from build123d import *

# Parameters (mm, degrees)
F0_W     = 10
F0_H     = 8
F1_DEPTH = 10
F2_T     = 1
F3_W     = 8
F3_H     = 2.908741124
F4_DEPTH = 0.1


with BuildPart() as f1:
    # F0 (on Top) → F1 (new body)
    with BuildSketch(Plane.XY):
        with Locations((-44.9863001704, 1.6067679121)):
            Rectangle(F0_W, F0_H)
    extrude(amount=F1_DEPTH)

    # F2
    f2_openings = [f1.faces().sort_by_distance(p)[0] for p in [
        (-44.9863, 1.606768, 10),
    ]]
    offset(amount=F2_T, openings=f2_openings, kind=Kind.INTERSECTION)

    # F3 (on face) → F4 (join)
    with BuildSketch(Plane.YZ.offset(-38.9863001704)):
        with Locations((1.6067679121, 6.545629438)):
            Rectangle(F3_W, F3_H)
    extrude(amount=F4_DEPTH)


solid = f1.part
For this review, take the finished solid that the model builds, in its own axes (mm). A direction names the side the tool comes from. Round coordinates to 2 decimals unless told otherwise and drop trailing zeros. Loops run counter-clockwise (first coordinate to the right, second up) from the corner with the lowest first, then second, coordinate; pieces in that order, holes last. Notation, with made-up numbers: (18, -24) - (25, -24) arc R20 cw to (25, 8) - close; hole circle Ø8 at (52, 35.5). An arc over 180 degrees is marked (long way). Use one line per item in the form item = value.
1) Mouldability with a two-part tool opening along Y and no side actions: class faces 3 (the face through (-39.986, 2, 5)), 4 (the face through (-50.986, 2, 4)), 5 (the face through (-45, 6.607, 4)) as pulls with the +Y half, pulls with the -Y half, needs draft (parallel to the pull), parting line crosses it, or undercut.
Solutions:
face_3 = undercut
face_4 = needs draft
face_5 = pulls with the +Y half
2) Clearance check with flat-ended pins moving along their axes: P1, Ø2, axis at x = -46, y = 2.5, coming from the +Z side; P2, Ø5, axis at y = 4, z = 2, coming from the +X side. State where each tip first meets the part, or that it passes through.
Solutions:
P1 = 0
P2 = -38.99
3) Wall thickness on probe 1 along Y at (x, z) = (-49, 5.25); probe 2 along X at (y, z) = (1.5, 2); probe 3 along X at (y, z) = (4, 6.25): over which ranges is each line inside the solid? List them lowest first.
Solutions:
probe_1 = -3.39 to -2.39, 5.61 to 6.61
probe_2 = -50.99 to -49.99, -39.99 to -38.99
probe_3 = -50.99 to -49.99, -39.99 to -38.89
4) We need section C-C on x = -43.5. Write out the cut boundary in (y, z), then the cut area to 3 significant figures.
Solutions:
outline = (-3.39, -1) - (6.61, -1) - (6.61, 10) - (5.61, 10) - (5.61, 0) - (-2.39, 0) - (-2.39, 10) - (-3.39, 10) - close
area = 30.0 mm2
5) We need section B-B on y = -1.5. Write out the cut boundary in (x, z), then the cut area to 3 significant figures.
Solutions:
outline = (-50.99, -1) - (-38.99, -1) - (-38.99, 5.09) - (-38.89, 5.09) - (-38.89, 8) - (-38.99, 8) - (-38.99, 10) - (-39.99, 10) - (-39.99, 0) - (-49.99, 0) - (-49.99, 10) - (-50.99, 10) - close
area = 32.3 mm2
6) We need section A-A on z = 8.5. Write out the cut boundary in (x, y).
Solutions:
outline = (-50.99, -3.39) - (-38.99, -3.39) - (-38.99, 6.61) - (-50.99, 6.61) - close; hole (-49.99, -2.39) - (-39.99, -2.39) - (-39.99, 5.61) - (-49.99, 5.61) - close
7) Tool access review of faces 1 (the face through (-45, -3.393, 4)), 2 (the face through (-49.986, 2, 5)): name each direction out of +Z, -Z, +X, -X, +Y, -Y from which nothing blocks a thin tool from reaching the whole face with its end or side.
Solutions:
face_1 = +Z, -Z, +X, -X, -Y
face_2 = +Z
